Design review of the part built by this model. Coordinates are the model's own, in mm. Face numbers are marked on the shaded views. A direction names the side the tool comes from. Coordinates: 2 decimals unless noted, no trailing zeros. Write each loop counter-clockwise with the first axis right and the second up, starting at its lowest first coordinate (ties: lowest second). Pieces come first, ordered by that corner, then holes. Notation, with made-up numbers: M -1,-21.5 L 55,-21.5 A28 cw 55,13.5 Z; hole C 18.25,36.5 d3. An arc over 180 degrees is marked long. One line per question, with ' | ' between items.
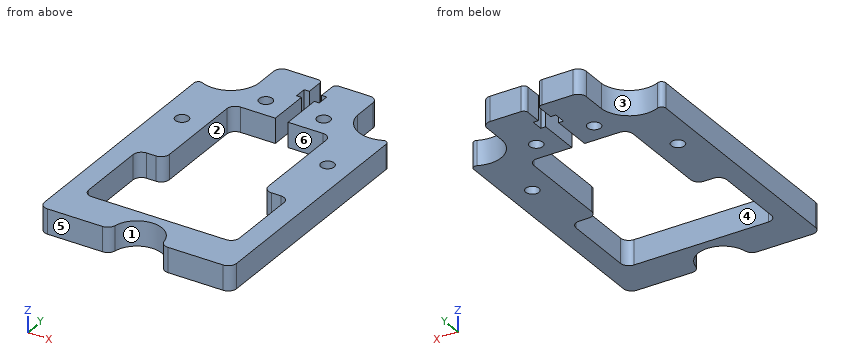
Autodesk Inventor part; units mm, degrees
ref_plane "YZ Plane" through (0, 0, 0) normal (1, 0, 0) x (0, 1, 0)
ref_plane "XZ Plane" through (0, 0, 0) normal (0, 1, 0) x (-1, 0, 0)
ref_plane "XY Plane" through (0, 0, 0) normal (0, 0, 1) x (1, 0, 0)
sketch "Sketch1" plane through (0, 0, 0) normal (0, 0, 1) x (1, 0, 0)
  line L0 (-11.9794, 21.8002) -> (-11.9794, -0.1998)
  line L1 (-13.9794, -2.1998) -> (-16.2294, -2.1998)
  line L2 (12.0206, -0.1998) -> (12.0206, 21.8002)
  line L3 (16.2706, -2.1998) -> (14.0206, -2.1998)
  line L4 (-23.2294, -2.1998) -> (-23.2294, 27.0455)
  line L5 (23.2706, -2.1998) -> (23.2706, 27.0455)
  line L6 (-1.5294, 33.8002) -> (-2.7294, 33.8002)
  line L7 (1.5706, 33.8002) -> (2.7706, 33.8002)
  arc A0 (12.0206, 33.8002) -> (21.8617, 27.958) centre (18.9993, 34.346) ccw
  arc A1 (-21.8205, 27.958) -> (-11.9794, 33.8002) centre (-18.9581, 34.346) ccw
  line L8 (-1.5294, 23.8002) -> (-1.5294, 33.8002)
  line L9 (1.5706, 23.8002) -> (1.5706, 33.8002)
  circle A2 centre (17.6456, 13.5013) radius 1.6
  circle A3 centre (-17.6044, 13.5013) radius 1.6
  circle A4 centre (7.0206, 28.8002) radius 1.6
  circle A5 centre (-6.9794, 28.8002) radius 1.6
  line L10 (-1.5294, 33.8002) -> (-2.7294, 33.8002)
  line L11 (2.7706, 33.8002) -> (2.7706, 36.7002)
  line L12 (-2.7294, 36.7002) -> (-2.7294, 33.8002)
  line L13 (-2.4794, 41.7002) -> (-9.9794, 41.7002)
  line L14 (-11.9794, 39.7002) -> (-11.9794, 33.8002)
  line L15 (12.0206, 33.8002) -> (12.0206, 39.7002)
  line L16 (10.0206, 41.7002) -> (2.5206, 41.7002)
  line L17 (1.5206, 36.7002) -> (1.5206, 40.7002)
  line L18 (-1.4794, 40.7002) -> (-1.4794, 36.7002)
  arc A6 (-9.9794, 23.8002) -> (-11.9794, 21.8002) centre (-9.9794, 21.8002) ccw
  arc A7 (12.0206, 21.8002) -> (10.0206, 23.8002) centre (10.0206, 21.8002) ccw
  arc A8 (12.0206, -0.1998) -> (14.0206, -2.1998) centre (14.0206, -0.1998) ccw
  arc A9 (-13.9794, -2.1998) -> (-11.9794, -0.1998) centre (-13.9794, -0.1998) ccw
  arc A10 (12.0206, 39.7002) -> (10.0206, 41.7002) centre (10.0206, 39.7002) ccw
  arc A11 (-9.9794, 41.7002) -> (-11.9794, 39.7002) centre (-9.9794, 39.7002) ccw
  arc A12 (-1.4794, 40.7002) -> (-2.4794, 41.7002) centre (-2.4794, 40.7002) ccw
  arc A13 (2.5206, 41.7002) -> (1.5206, 40.7002) centre (2.5206, 40.7002) ccw
  arc A14 (23.2706, 27.0455) -> (21.8617, 27.958) centre (22.2706, 27.0455) ccw
  arc A15 (-21.8205, 27.958) -> (-23.2294, 27.0455) centre (-22.2294, 27.0455) ccw
  line L19 (-23.2294, -2.1998) -> (-23.2294, -30.1998)
  line L20 (-21.2294, -32.1998) -> (21.2706, -32.1998)
  line L21 (23.2706, -30.1998) -> (23.2706, -2.1998)
  line L22 (-18.2294, -4.1998) -> (-18.2294, -21.1998)
  line L23 (18.2706, -4.1998) -> (18.2706, -21.1998)
  line L24 (16.2706, -23.1998) -> (-16.2294, -23.1998)
  arc A16 (-18.2294, -21.1998) -> (-16.2294, -23.1998) centre (-16.2294, -21.1998) ccw
  arc A17 (16.2706, -23.1998) -> (18.2706, -21.1998) centre (16.2706, -21.1998) ccw
  arc A18 (18.2706, -4.1998) -> (16.2706, -2.1998) centre (16.2706, -4.1998) ccw
  arc A19 (-16.2294, -2.1998) -> (-18.2294, -4.1998) centre (-16.2294, -4.1998) ccw
  arc A20 (21.2706, -32.1998) -> (23.2706, -30.1998) centre (21.2706, -30.1998) ccw
  arc A21 (-23.2294, -30.1998) -> (-21.2294, -32.1998) centre (-21.2294, -30.1998) ccw
  line L25 (10.0206, 23.8002) -> (1.5706, 23.8002)
  line L26 (-1.5294, 23.8002) -> (-9.9794, 23.8002)
  line L27 (-2.7294, 33.8002) -> (-1.5294, 33.8002)
  line L28 (1.5706, 33.8002) -> (2.7706, 33.8002)
  line L29 (2.7706, 36.7002) -> (1.5206, 36.7002)
  line L30 (-1.4794, 36.7002) -> (-2.7294, 36.7002)
  point P0 (0, 0)
  point P1 (0, 0)
  point P2 (-23.2294, 28.8002)
  point P3 (23.2706, 28.8002)
  point P4 (-23.2294, -32.1998)
  point P5 (-18.2294, -23.1998)
  dimension "d0" = 31
  dimension "d1" = 7
  dimension "d2" = 7
  dimension "d6" = 2
  dimension "d8" = 30
  dimension "d13" = 2
extrude "Extrusion1" add sketch "Sketch1" along normal blind 6
sketch "Sketch2" plane through (0, 0, 6) normal (0, 0, 1) x (1, 0, 0)
  line L0 (-21.2294, -32.1998) -> (21.2706, -32.1998)
  line L1 (0.0206, -32.1998) -> (0.0206, -28.1998)
  line L2 (0.0206, -28.1998) -> (0.0206, -34.998)
  line L3 (0.0206, -34.998) -> (0.0206, -28.1998)
  circle A0 centre (0.0206, -31.5989) radius 5.0514
  circle A1 centre (0.0206, -31.5989) radius 6.0346
  point P0 (0, 0)
  dimension "d16" = 4
extrude "Extrusion2" cut sketch "Sketch2" against normal blind 6
fillet "Fillet1" radius 2 2 edges at (6.0253, -32.1998, 3) (-5.984, -32.1998, 3)
properties part number "Hotend Slide Part 2" material "Acetal Resin, White"
1. Take a section at A-A (y = -16). Write out the cut boundary in (x, z).
Answer sheet:
outline: M -23.23,0 L -18.23,0 L -18.23,6 L -23.23,6 Z; M 18.27,0 L 23.27,0 L 23.27,6 L 18.27,6 Z
2. Insertion check: pin 1 Ø1 at (x, z) = (-2, 3.5) entering from -Y; pin 2 Ø1 at (x, z) = (2, 4) entering from +Y; pin 3 Ø3 at (y, z) = (35.5, 2.5) entering from +X; pin 4 Ø3 at (y, z) = (35.5, 2) entering from -X. Each pin has a flat end and moves straight along its axis. Give the tip position at first contact, or say it passes through.
Answer sheet:
pin 1: y = -26.12 | pin 2: y = 41.7 | pin 3: x = 12.02 | pin 4: x = -11.98
3. Draft analysis for pull direction Y (two halves, no side actions). For the marked faces 3, 4, 5 and 6, state which applies: pulls with the +Y half, pulls with the -Y half, needs draft (parallel to the pull), parting line crosses it, or undercut.
Answer sheet:
face 3: pulls with the +Y half | face 4: undercut | face 5: pulls with the -Y half | face 6: undercut
4. Take a section at B-B (y = 18). Write out the cut boundary in (x, z).
Answer sheet:
outline: M -23.23,0 L -11.98,0 L -11.98,6 L -23.23,6 Z; M 12.02,0 L 23.27,0 L 23.27,6 L 12.02,6 Z
5. Tool access review of the marked faces 1 and 2: name each direction out of +Z, -Z, +X, -X, +Y, -Y from which nothing blocks a thin tool from reaching the whole face with its end or side.
Answer sheet:
face 1: +Z, -Z, -Y | face 2: +Z, -Z
6. Take a section at D-D (x = 0). Write out the cut boundary in (y, z), then the cut area to 3 significant figures.
Answer sheet:
outline: M -25.56,0 L -23.2,0 L -23.2,6 L -25.56,6 Z | area: 14.2 mm^2
7. Take a section at C-C (z = 1.95). Count the separate pieces of the cut face and the enclosed holes in it, then the cut area to 3 significant figures.
Answer sheet:
separate pieces: 1 | enclosed holes: 4 | area: 1,590 mm^2
8. To check wall thickness, follow line 1 along X through (y, z) = (38, 4.2); line 2 along Y through (x, z) = (9, 4.95); line 3 along X through (y, z) = (22, 5.15). State the ranges of each line that lie inside material, in increasing order. Write a range as [from, to].
Answer sheet:
line 1: [-11.98, -1.48], [1.52, 12.02] | line 2: [-32.2, -23.2], [23.8, 41.7] | line 3: [-23.23, -11.97], [12.01, 23.27]
